CAD build for the part. Positions are in the model's coordinates, mm. A direction names the side the tool comes from. Round coordinates to 2 decimals unless told otherwise and drop trailing zeros. Loops run counter-clockwise (first coordinate to the right, second up) from the corner with the lowest first, then second, coordinate; pieces in that order, holes last. Notation, with made-up numbers: M 1,23.5 L 51,23.5 A25 ccw 51,35.5 Z; hole C 53,58 d6. An arc over 180 degrees is marked long. One line per item, written item: value. Start each with the question number.
from build123d import *

# Parameters (mm, degrees)
SKETCH1_R           = 7.65
SKETCH1_W           = 17.157732918
SKETCH1_H           = 9
SKETCH1_W_2         = 8
SKETCH1_H_2         = 3
BOSS_EXTRUDE1_DEPTH = 1.5


with BuildPart() as part:
    # Sketch1 → Boss-Extrude1 (new body, symmetric)
    with BuildSketch(Plane(origin=(0, 0, 0), x_dir=(1, 0, 0), z_dir=(0, 1, 0))):
        with BuildLine():
            Line((-16.842384682, 9.84807753), (-18.578866459, 0))
            Line((-18.578866459, 0), (-8.578866459, 0))
            Line((-8.578866459, 0), (8.578866459, 0))
            Line((8.578866459, 0), (18.578866459, 0))
            Line((18.578866459, 0), (16.842384682, 9.84807753))
            Line((16.842384682, 9.84807753), (13.887961423, 9.327132997))
            Line((13.887961423, 9.327132997), (11.682629567, 21.83419146))
            Line((11.682629567, 21.83419146), (14.637052826, 22.355135993))
            Line((14.637052826, 22.355135993), (14.427433582, 23.543945803))
            ThreePointArc((14.427433582, 23.543945803), (0, 35.65), (-14.427433582, 23.543945803))
            Line((-14.427433582, 23.543945803), (-14.637052826, 22.355135993))
            Line((-14.637052826, 22.355135993), (-11.682629567, 21.83419146))
            Line((-11.682629567, 21.83419146), (-13.887961423, 9.327132997))
            Line((-13.887961423, 9.327132997), (-16.842384682, 9.84807753))
        make_face()
        with Locations((0, 21)):
            Circle(SKETCH1_R, mode=Mode.SUBTRACT)
        with Locations((0, -4.5)):
            Rectangle(SKETCH1_W, SKETCH1_H)
        with Locations((0, -4.5)):
            Rectangle(SKETCH1_W_2, SKETCH1_H_2, mode=Mode.SUBTRACT)
    extrude(amount=BOSS_EXTRUDE1_DEPTH, both=True)


solid = part.part
(1) Slice it at D-D, the plane x = 6.5. List the corners of the cut face in (y, z).
(2) Slice it at A-A, the plane x = 0. List the corners of the cut face in (y, z).
(3) Flat gauge pins, fed straight in: P1, Ø1.5, axis at y = 0.5, z = -25, coming from the -X side; P2, Ø1.5, axis at y = -0.5, z = 5, coming from the -X side; P3, Ø1, axis at y = -0.5, z = -10.5, coming from the -X side. Where does each tip first touch, or does it go through?
(4) Probe L1, parallel to Z at x = -1.5, y = -1.4; L2, parallel to Z at x = -0.5, y = 0.7; L3, parallel to X at y = 0.75, z = -21. List the from-to ranges inside material, lowest first.
(5) Mould opens along Z. For faces 1 (the flat face through (8.579, 0, 5)), 2 (the flat face through (14.534, 0.021, -22.941)), 3 (the flat face through (12.8, 0, -15.5)) say: pulls with the +Z half, pulls with the -Z half, needs draft (parallel to the pull), parting line crosses it, or undercut.
(6) Which spindle directions (+Z, -Z, +X, -X, +Y, -Y) get a long thin tool onto all of the face, cutting with end or side? Do faces 4 (the flat face through (-13.2, 0, -22.1)), 5 (the flat face through (-8.579, 0, 5)), 6 (the flat face through (0, 0, 3)). Say none if no direction does.
(7) Slice it at B-B, the plane y = 0.15. List the corners of the cut face in (x, z).
(8) Slice it at C-C, the plane z = -21. List the corners of the cut face in (x, y), and give its area (3 significant figures).
Check result:
1. outline: M -1.5,-34.13 L 1.5,-34.13 L 1.5,-25.03 L -1.5,-25.03 Z; M -1.5,-16.97 L 1.5,-16.97 L 1.5,9 L -1.5,9 Z
2. outline: M -1.5,-35.65 L 1.5,-35.65 L 1.5,-28.65 L -1.5,-28.65 Z; M -1.5,-13.35 L 1.5,-13.35 L 1.5,3 L -1.5,3 Z; M -1.5,6 L 1.5,6 L 1.5,9 L -1.5,9 Z
3. P1: stops at x = -14.28
3. P2: stops at x = -8.58
3. P3: stops at x = -13.77
4. L1: z = -35.57 to -28.5, -13.5 to 3, 6 to 9
4. L2: z = -35.64 to -28.63, -13.37 to 3, 6 to 9
4. L3: x = -11.83 to -7.65, 7.65 to 11.83
5. face 1: needs draft
5. face 2: pulls with the -Z half
5. face 3: undercut
6. face 4: -X, +Y, -Y
6. face 5: +Z, -X, +Y, -Y
6. face 6: +Y, -Y
7. outline: M -18.58,0 L -16.84,-9.85 L -13.89,-9.33 L -11.68,-21.83 L -14.64,-22.36 L -14.43,-23.54 A14.65 ccw 14.43,-23.54 L 14.64,-22.36 L 11.68,-21.83 L 13.89,-9.33 L 16.84,-9.85 L 18.58,0 L 8.58,0 L 8.58,9 L -8.58,9 L -8.58,0 Z; hole C 0,-21 d15.3; hole M -4,3 L 4,3 L 4,6 L -4,6 Z
8. outline: M -11.83,-1.5 L -7.65,-1.5 L -7.65,1.5 L -11.83,1.5 Z; M 7.65,-1.5 L 11.83,-1.5 L 11.83,1.5 L 7.65,1.5 Z
8. area: 25.1 mm^2
